from build123d import *

# Parameters (mm, degrees)
ESBO_O1_W                  = 30
ESBO_O1_H                  = 10
RESSALTO_EXTRUS_O1_DEPTH   = 59
RESSALTO_EXTRUS_O1_2_DEPTH = 59
ESBO_O2_W                  = 30
ESBO_O2_H                  = 42
RESSALTO_EXTRUS_O2_DEPTH   = 8
CORTE_EXTRUS_O1_DEPTH      = 31
CORTE_EXTRUS_O2_DEPTH      = 4
FILETE1_R                  = 4
ESBO_O5_R                  = 4
CORTE_EXTRUS_O3_DEPTH      = 60
FILETE2_R                  = 6


with BuildPart() as part:
    # Esbo_o1 → Ressalto-extrus_o1 (new body)
    with BuildSketch(Plane.XY):
        with Locations((0, 26)):
            Rectangle(ESBO_O1_W, ESBO_O1_H)
    extrude(amount=RESSALTO_EXTRUS_O1_DEPTH)



with BuildPart() as body_2:
    # Esbo_o1 → Ressalto-extrus_o1 2 (new body)
    with BuildSketch(Plane.XY):
        with Locations((0, -26)):
            Rectangle(ESBO_O1_W, ESBO_O1_H)
    extrude(amount=RESSALTO_EXTRUS_O1_2_DEPTH)


with BuildPart() as part_1:
    add(part.part)

    add(body_2.part)  # Ressalto-extrus_o2 merges body 2
    # Esbo_o2 → Ressalto-extrus_o2 (add)
    with BuildSketch(Plane(origin=(0, 0, 0), x_dir=(-1, 0, 0), z_dir=(0, 0, -1))):
        Rectangle(ESBO_O2_W, ESBO_O2_H)
    extrude(amount=-RESSALTO_EXTRUS_O2_DEPTH)

    # Esbo_o3 → Corte-extrus_o1 (cut, through all)
    with BuildSketch(Plane.ZY.offset(15)):
        with BuildLine():
            Line((34.464319348, 27.180824333), (34.464319348, 21))
            Line((34.464319348, 21), (52.664319348, 21))
            Line((52.664319348, 21), (52.664319348, 27.13384671))
            ThreePointArc((52.664319348, 27.13384671), (52.473932816, 27.593480457), (52.014299068, 27.783866989))
            Line((52.014299068, 27.783866989), (48.83365389, 27.783866989))
            Line((48.83365389, 27.783866989), (48.853388433, 27.775806736))
            Line((48.853388433, 27.775806736), (48.83365389, 27.775908805))
            Line((48.83365389, 27.775908805), (48.83365389, 27.124623249))
            ThreePointArc((48.83365389, 27.124623249), (48.064319348, 22.760238146), (47.294984805, 27.124623249))
            Line((47.294984805, 27.124623249), (47.294984805, 27.783866989))
            Line((47.294984805, 27.783866989), (40.021105511, 27.821488377))
            Line((40.021105511, 27.821488377), (39.721105511, 27.821488377))
            Line((39.721105511, 27.821488377), (39.721105511, 27.162244637))
            ThreePointArc((39.721105511, 27.162244637), (39.064319348, 22.760238146), (38.407533184, 27.162244637))
            Line((38.407533184, 27.162244637), (38.407533184, 27.821488377))
            Line((38.407533184, 27.821488377), (35.104983392, 27.821488377))
            ThreePointArc((35.104983392, 27.821488377), (34.654639493, 27.631168232), (34.464319348, 27.180824333))
        make_face()
        with BuildLine():
            ThreePointArc((51.8897547, -26.423845407), (52.437454615, -26.196980674), (52.664319348, -25.649280759))
            Line((52.664319348, -25.649280759), (52.664319348, -20.77))
            Line((52.664319348, -20.77), (34.5, -20.77))
            Line((34.5, -20.77), (34.464319348, -20.770417185))
            Line((34.464319348, -20.770417185), (34.464319348, -25.649280759))
            ThreePointArc((34.464319348, -25.649280759), (34.69118408, -26.196980674), (35.238883995, -26.423845407))
            Line((35.238883995, -26.423845407), (38.294984805, -26.423845407))
            Line((38.294984805, -26.423845407), (38.294984805, -25.584623249))
            ThreePointArc((38.294984805, -25.584623249), (39.064319348, -21.220238146), (39.83365389, -25.584623249))
            Line((39.83365389, -25.584623249), (39.83365389, -26.423845407))
            Line((39.83365389, -26.423845407), (47.294984805, -26.423845407))
            Line((47.294984805, -26.423845407), (47.294984805, -25.584623249))
            ThreePointArc((47.294984805, -25.584623249), (48.064319348, -21.220238146), (48.83365389, -25.584623249))
            Line((48.83365389, -25.584623249), (48.83365389, -26.423845407))
            Line((48.83365389, -26.423845407), (51.8897547, -26.423845407))
        make_face()
    extrude(amount=-CORTE_EXTRUS_O1_DEPTH, mode=Mode.SUBTRACT)

    # Esbo_o4 → Corte-extrus_o2 (cut)
    with BuildSketch(Plane.ZY.offset(15)):
        with BuildLine():
            Line((47.294984805, 27.783866989), (48.853388433, 27.775806736))
            Line((48.853388433, 27.775806736), (48.853388433, 27.117338044))
            ThreePointArc((48.853388433, 27.117338044), (48.055619332, 22.760254966), (47.291568671, 27.123377136))
            Line((47.291568671, 27.123377136), (47.294984805, 27.783866989))
        make_face()
        with BuildLine():
            Line((38.407533184, 27.821488377), (38.407533184, 27.162244637))
            ThreePointArc((38.407533184, 27.162244637), (39.064319348, 22.760238146), (39.721105511, 27.162244637))
            Line((39.721105511, 27.162244637), (39.721105511, 27.821488377))
            Line((39.721105511, 27.821488377), (38.407533184, 27.821488377))
        make_face()
    extrude(amount=-CORTE_EXTRUS_O2_DEPTH, mode=Mode.SUBTRACT)

    # Filete1
    filete1_edges = [part_1.edges().sort_by_distance(p)[0] for p in [
        (0, 21, 8),
        (0, -21, 8),
    ]]
    fillet(filete1_edges, radius=FILETE1_R)

    # Esbo_o5 → Corte-extrus_o3 (cut, through all)
    with BuildSketch(Plane(origin=(0, 0, 0), x_dir=(-1, 0, 0), z_dir=(0, 0, -1))):
        with Locations((0, -12)):
            Circle(ESBO_O5_R)
        with Locations((0, 12)):
            Circle(ESBO_O5_R)
    extrude(amount=-CORTE_EXTRUS_O3_DEPTH, mode=Mode.SUBTRACT)

    # Filete2
    filete2_edges = [part_1.edges().sort_by_distance(p)[0] for p in [
        (0, -31, 0),
        (0, 31, 0),
    ]]
    fillet(filete2_edges, radius=FILETE2_R)


solid = part_1.part
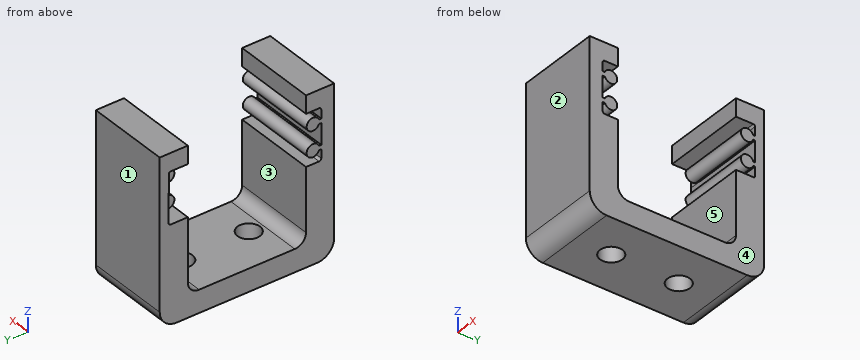
The model under review builds one solid part; all positions refer to its coordinate system, in mm. Face numbers are marked on the shaded views. A direction names the side the tool comes from. Coordinates: 2 decimals unless noted, no trailing zeros. Write each loop counter-clockwise with the first axis right and the second up, starting at its lowest first coordinate (ties: lowest second). Pieces come first, ordered by that corner, then holes. Notation, with made-up numbers: (-38.75, 66) -> (8.25, 66) arc R29 ccw to (8.25, 104) -> close; hole circle Ø5 at (38, 85.5). An arc over 180 degrees is marked (long way). Answer in a Markdown table with one row per item.
1. We need section C-C, the plane x = 0. Give the number of separate pieces and of enclosed holes in the cut face, and give its area (3 significant figures).
Answers below:
| item | result |
|---|---|
| separate pieces | 3 |
| enclosed holes | 0 |
| area | 1,220 mm^2 |
2. Draft analysis for pull direction Y (two halves, no side actions). For the marked faces 1, 2 and 3, state which applies: +Y half, -Y half, draft (parallel to the pull), parting line (faces both ways), or undercut.
Answers below:
| item | result |
|---|---|
| face 1 | +Y half |
| face 2 | -Y half |
| face 3 | undercut |
3. We need section D-D, the plane y = 24. State the section outline as (x, z) points.
Answers below:
| item | result |
|---|---|
| outline | (-15, 0) -> (15, 0) -> (15, 34.46) -> (-15, 34.46) -> close; (-15, 52.66) -> (15, 52.66) -> (15, 59) -> (-15, 59) -> close; (-11, 37.05) -> (15, 37.05) -> (15, 41.07) -> (-11, 41.07) -> close; (-11, 46.05) -> (15, 46.05) -> (15, 50.07) -> (-11, 50.07) -> close |
4. Clearance check with flat-ended pins moving along their axes: pin 1 Ø1.4 at (y, z) = (25, 40) entering from -X; pin 2 Ø0.5 at (x, y) = (8.5, 27.5) entering from -Z; pin 3 Ø6 at (x, y) = (-3, 0) entering from +Z. State where each tip first meets the part, or that it passes through.
Answers below:
| item | result |
|---|---|
| pin 1 | stops at x = -11 |
| pin 2 | stops at z = 0.44 |
| pin 3 | stops at z = 8 |
5. We need section B-B, the plane y = -12. State the section outline as (x, z) points.
Answers below:
| item | result |
|---|---|
| outline | (-15, 0) -> (-4, 0) -> (-4, 8) -> (-15, 8) -> close; (4, 0) -> (15, 0) -> (15, 8) -> (4, 8) -> close |
6. For the marked faces 4 and 5, list the 3-axis set-ups (+Z, -Z, +X, -X, +Y, -Y) from which the entire face can be reached by the end or side of a thin tool; tool diameter is ignored.
Answers below:
| item | result |
|---|---|
| face 4 | +Z, -Z, +X, +Y, -Y |
| face 5 | +Z, +X, -X |
7. We need section A-A, the plane z = 18.5. State the section outline as (x, y) points, and give its area (3 significant figures).
Answers below:
| item | result |
|---|---|
| outline | (-15, -31) -> (15, -31) -> (15, -21) -> (-15, -21) -> close; (-15, 21) -> (15, 21) -> (15, 31) -> (-15, 31) -> close |
| area | 600 mm^2 |
8. Wall thickness on probe 1 along Y at (x, z) = (0, 6); probe 2 along Z at (x, y) = (0.5, 22); probe 3 along Y at (x, z) = (-5.5, 42): over which ranges is each line inside the solid? List them lowest first. Write a range as [from, to].
Answers below:
| item | result |
|---|---|
| probe 1 | y = [-31, -16], [-8, 8], [16, 31] |
| probe 2 | z = [0, 34.46], [52.66, 59] |
| probe 3 | y = [-31, -26.42], [27.81, 31] |
